```python
from build123d import *

# Parameters (mm, degrees)
SKETCH1_W           = 144
SKETCH1_H           = 35.5
BOSS_EXTRUDE1_DEPTH = 3
FILLET1_R           = 2
SKETCH2_W           = 3
SKETCH2_H           = 18
CUT_EXTRUDE1_DEPTH  = 3
BOSS_EXTRUDE2_DEPTH = 3


with BuildPart() as part:
    # Sketch1 → Boss-Extrude1 (new body)
    with BuildSketch(Plane(origin=(0, 0, 0), x_dir=(0, 0, -1), z_dir=(1, 0, 0))):
        Rectangle(SKETCH1_W, SKETCH1_H)
    extrude(amount=BOSS_EXTRUDE1_DEPTH)

    # Fillet1
    fillet1_edges = [part.edges().sort_by_distance(p)[0] for p in [
        (1.5, 17.75, 72),
        (1.5, 17.75, -72),
    ]]
    fillet(fillet1_edges, radius=FILLET1_R)

    # Sketch2 → Cut-Extrude1 (cut)
    with BuildSketch(Plane(origin=(3, 0, 0), x_dir=(0, 0, -1), z_dir=(1, 0, 0))):
        with Locations((-40.5, -8.75)):
            Rectangle(SKETCH2_W, SKETCH2_H)
        with Locations((40.5, -8.75)):
            Rectangle(SKETCH2_W, SKETCH2_H)
    extrude(amount=-CUT_EXTRUDE1_DEPTH, mode=Mode.SUBTRACT)

    # Sketch3 → Boss-Extrude2 (add)
    with BuildSketch(Plane(origin=(3, 0, 0), x_dir=(0, 0, -1), z_dir=(1, 0, 0))):
        Polygon((-72, -17.75), (-72, -27.75), (-42, -17.75), align=None)
    boss_extrude2 = extrude(amount=-BOSS_EXTRUDE2_DEPTH)

    # Mirror1: Boss-Extrude2 across plane
    add(boss_extrude2.mirror(Plane.XY))


solid = part.part
```
Source: CAD feature listing. Evaluate the final solid. Frame: model axes, mm. A direction names the side the tool comes from. Round coordinates to 2 decimals unless told otherwise and drop trailing zeros. Loops run counter-clockwise (first coordinate to the right, second up) from the corner with the lowest first, then second, coordinate; pieces in that order, holes last.
1. Mould query, pull axis Z, two halves, no side actions, for faces 1 (the flat face through (2, -9, 42)), 2 (the flat face through (2, -6, -72)), 3 (the flat face through (3, 0, -1)). Classes: released by +Z, released by -Z, zero draft, split by the parting line, or undercut.
2. Contact query for flat-ended pins moving along their axis: pin 1 (1.5 mm diameter, centred on x = 1.5, z = -16.5, fed in from -Y); pin 2 (0.9 mm diameter, centred on x = 2, z = -41, fed in from -Y). Output: stop coordinate, or through.
3. Ray query, L1, parallel to Z at x = 2.35, y = -10; L2, parallel to Y at x = 2.5, z = 22; L3, parallel to Y at x = 2, z = -56. Return the intervals inside material, ascending.
4. Section query B-B on x = 0.85. Output: boundary loops of the cut face in (y, z).
5. Section query C-C on z = 34. Output: boundary loops of the cut face in (x, y), and give its area (4 significant figures).
6. Access query for faces 4 (the flat face through (0, 0, -1)), 5 (the flat face through (1.52, -22.82, 57.21)). Directions: +Z, -Z, +X, -X, +Y, -Y. A direction counts if a zero-diameter tool reaches every point of the face in a straight line with its end or side. Return the directions, or none.
7. Section query A-A on y = -3. Output: boundary loops of the cut face in (x, z).
Answers below:
1. face 1: undercut
1. face 2: released by -Z
1. face 3: zero draft
2. pin 1: stops at y = -17.75
2. pin 2: stops at y = 0.25
3. L1: z = -72 to -42, -39 to 39, 42 to 72
3. L2: y = -17.75 to 17.75
3. L3: y = -22.42 to 17.75
4. outline: (-27.75, -72) - (15.75, -72) arc R2 ccw to (17.75, -70) - (17.75, 70) arc R2 ccw to (15.75, 72) - (-27.75, 72) - (-17.75, 42) - (0.25, 42) - (0.25, 39) - (-17.75, 39) - (-17.75, -39) - (0.25, -39) - (0.25, -42) - (-17.75, -42) - close
5. outline: (0, -17.75) - (3, -17.75) - (3, 17.75) - (0, 17.75) - close
5. area: 106.5 mm2
6. face 4: +Z, -Z, -X, +Y, -Y
6. face 5: +X, -X, -Y
7. outline: (0, -72) - (3, -72) - (3, -42) - (0, -42) - close; (0, -39) - (3, -39) - (3, 39) - (0, 39) - close; (0, 42) - (3, 42) - (3, 72) - (0, 72) - close
